```python
from build123d import *

# Parameters (mm, degrees)
SKETCH1_R           = 7.5
BOSS_EXTRUDE1_DEPTH = 200
SKETCH2_R           = 45
BOSS_EXTRUDE2_DEPTH = 10


with BuildPart() as part:
    # Sketch1 → Boss-Extrude1 (new body, symmetric)
    with BuildSketch(Plane(origin=(0, 0, 0), x_dir=(0, 0, -1), z_dir=(1, 0, 0))):
        Circle(SKETCH1_R)
    extrude(amount=BOSS_EXTRUDE1_DEPTH, both=True)

    # Sketch2 → Boss-Extrude2 (add)
    with BuildSketch(Plane(origin=(200, 0, 0), x_dir=(0, 0, -1), z_dir=(1, 0, 0))):
        Circle(SKETCH2_R)
    boss_extrude2 = extrude(amount=BOSS_EXTRUDE2_DEPTH)

    # Mirror1: Boss-Extrude2 across plane
    add(boss_extrude2.mirror(Plane(origin=(0, 0, 0), x_dir=(0, 0, 1), z_dir=(1, 0, 0))))


solid = part.part
```
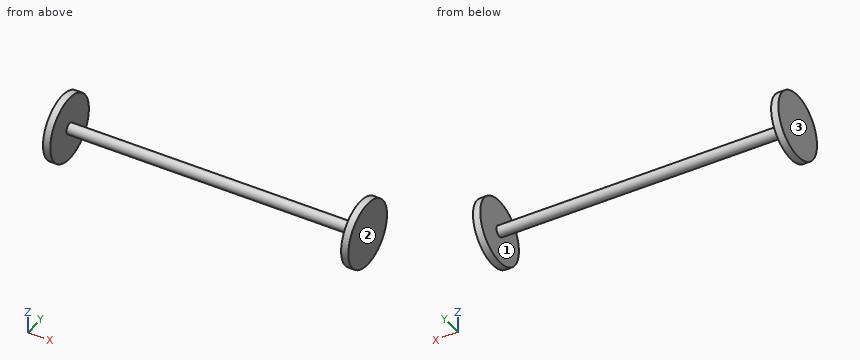
For this review, take the finished solid that the model builds, in its own axes (mm). Face numbers are marked on the shaded views. Coordinates: 2 decimals unless noted, no trailing zeros. Write each loop counter-clockwise with the first axis right and the second up, starting at its lowest first coordinate (ties: lowest second). Pieces come first, ordered by that corner, then holes. Notation, with made-up numbers: (9, 53.25) - (46, 53.25) arc R27 cw to (46, 87.25) - close; hole circle Ø5 at (-24.5, -12.5). An arc over 180 degrees is marked (long way). Answer in a Markdown table with one row per item. Add a question column.
Q1. We need section C-C, the plane y = 18.5. State the section outline as (x, z) points.
Q2. We need section A-A, the plane y = 0. State the section outline as (x, z) points, and give its area (3 significant figures).
Q3. For probe 1 along X at (y, z) = (-18.5, 13); probe 2 along Z at (x, y) = (-163.5, 4); probe 3 along Y at (x, z) = (-168, 2), list the stretches that pass through material, from the lowest coordinate up.
Q4. We need section B-B, the plane z = -18. State the section outline as (x, y) points, and give its area (3 significant figures).
Q5. Draft analysis for pull direction X (two halves, no side actions). For the marked faces 1, 2 and 3, state which applies: +X half, -X half, draft (parallel to the pull), parting line (faces both ways), or undercut.
Q6. For P1, Ø1, axis at x = 26.5, z = 3.5, coming from the +Y side; P2, Ø6, axis at x = 21, z = -6, coming from the -Y side, all flat-tipped, find the tip position at first contact; note any pin that passes through.
Answer list:
| question | item | result |
|---|---|---|
| 1 | outline | (-210, -41.02) - (-200, -41.02) - (-200, 41.02) - (-210, 41.02) - close; (200, -41.02) - (210, -41.02) - (210, 41.02) - (200, 41.02) - close |
| 2 | outline | (-210, -45) - (-200, -45) - (-200, -7.5) - (200, -7.5) - (200, -45) - (210, -45) - (210, 45) - (200, 45) - (200, 7.5) - (-200, 7.5) - (-200, 45) - (-210, 45) - close |
| 2 | area | 7,800 mm2 |
| 3 | probe 1 | x = -210 to -200, 200 to 210 |
| 3 | probe 2 | z = -6.34 to 6.34 |
| 3 | probe 3 | y = -7.23 to 7.23 |
| 4 | outline | (-210, -41.24) - (-200, -41.24) - (-200, 41.24) - (-210, 41.24) - close; (200, -41.24) - (210, -41.24) - (210, 41.24) - (200, 41.24) - close |
| 4 | area | 1,650 mm2 |
| 5 | face 1 | undercut |
| 5 | face 2 | +X half |
| 5 | face 3 | -X half |
| 6 | P1 | stops at y = 6.87 |
| 6 | P2 | stops at y = -6.87 |
